from build123d import *

# Parameters (mm, degrees)
SKETCH1_W           = 55
SKETCH1_H           = 22
BOSS_EXTRUDE1_DEPTH = 18
CUT_EXTRUDE2_START  = -55
CUT_EXTRUDE2_DEPTH  = 55
SKETCH5_W           = 50
SKETCH5_H           = 17
CUT_EXTRUDE3_DEPTH  = 10
FILLET1_R           = 2.5
CUT_EXTRUDE4_DEPTH  = 3
SKETCH8_W           = 5.5
SKETCH8_H           = 1.5
CUT_EXTRUDE5_DEPTH  = 32


# Read off the part's stored shape, not the designer's step: Cut-Extrude2
with BuildPart() as part:
    # Sketch1 → Boss-Extrude1 (new body)
    with BuildSketch(Plane.XY):
        with Locations((-16.417297699, 9.516109874)):
            Rectangle(SKETCH1_W, SKETCH1_H)
    extrude(amount=BOSS_EXTRUDE1_DEPTH)

    # Cut-Extrude2 outline → Cut-Extrude2 (cut)
    with BuildSketch(Plane(origin=(11.082702301, 0, 0), x_dir=(0, 0, -1), z_dir=(1, 0, 0)).offset(CUT_EXTRUDE2_START)):
        with BuildLine():
            add(Edge.make_bspline(
                [(0, 1.8942341), (-9.999457611, 9.516109874), (0, 17.137985647)],
                knots=[0, 0, 0, 1, 1, 1], degree=2))
            Line((0, 1.8942341), (0, 17.137985647))
        make_face()
    extrude(amount=CUT_EXTRUDE2_DEPTH, mode=Mode.SUBTRACT)

    # Sketch5 → Cut-Extrude3 (cut)
    with BuildSketch(Plane(origin=(0, 0, 0), x_dir=(-1, 0, 0), z_dir=(0, 0, -1))):
        with Locations((16.417297699, 9.516109874)):
            Rectangle(SKETCH5_W, SKETCH5_H)
    extrude(amount=-CUT_EXTRUDE3_DEPTH, mode=Mode.SUBTRACT)

    # Fillet1
    fillet1_edges = [part.edges().sort_by_distance(p)[0] for p in [
        (11.082702301, 9.516109874, 18),
        (-16.417297699, 20.516109874, 18),
        (-43.917297699, 9.516109874, 18),
        (-16.417297699, -1.483890126, 18),
    ]]
    fillet(fillet1_edges, radius=FILLET1_R)

    # Sketch7 → Cut-Extrude4 (cut)
    with BuildSketch(Plane.XY.offset(18)):
        with BuildLine():
            Line((-39.308664902, 14.016109874), (-20.917297699, 14.016109874))
            Line((-20.917297699, 14.016109874), (-20.917297699, 18.016109874))
            ThreePointArc((-20.917297699, 18.016109874), (-16.417297699, 22.516109874), (-11.917297699, 18.016109874))
            Line((-11.917297699, 18.016109874), (-11.917297699, 14.016109874))
            Line((-11.917297699, 14.016109874), (6.474069505, 14.016109874))
            ThreePointArc((6.474069505, 14.016109874), (10.974069505, 9.516109874), (6.474069505, 5.016109874))
            Line((6.474069505, 5.016109874), (-11.917297699, 5.016109874))
            Line((-11.917297699, 5.016109874), (-11.917297699, 1.016109874))
            ThreePointArc((-11.917297699, 1.016109874), (-16.417297699, -3.483890126), (-20.917297699, 1.016109874))
            Line((-20.917297699, 1.016109874), (-20.917297699, 5.016109874))
            Line((-20.917297699, 5.016109874), (-39.308664902, 5.016109874))
            ThreePointArc((-39.308664902, 5.016109874), (-43.808664902, 9.516109874), (-39.308664902, 14.016109874))
        make_face()
    extrude(amount=-CUT_EXTRUDE4_DEPTH, mode=Mode.SUBTRACT)

    # Sketch8 → Cut-Extrude5 (cut)
    with BuildSketch(Plane(origin=(0, 20.516109874, 0), x_dir=(1, 0, 0), z_dir=(0, 1, 0))):
        with Locations((-37.042297699, -13.165280764)):
            Rectangle(SKETCH8_W, SKETCH8_H)
        with Locations((-7.250631032, -13.165280764)):
            Rectangle(SKETCH8_W, SKETCH8_H)
        with Locations((4.207702301, -13.165280764)):
            Rectangle(SKETCH8_W, SKETCH8_H)
        with Locations((-25.583964365, -13.165280764)):
            Rectangle(SKETCH8_W, SKETCH8_H)
    extrude(amount=-CUT_EXTRUDE5_DEPTH, mode=Mode.SUBTRACT)


solid = part.part
Could you check a few things on this model? Use its own coordinates, in mm. A direction names the side the tool comes from. Give positions to 0.01 mm unless a question says otherwise; leave off trailing zeros. Order: outer loops, then holes, each group sorted by start corner. A loop starts at its lowest first (then second) coordinate and runs counter-clockwise, first axis right, second up.
1. Thinking about a two-plate mould opening in X: for faces 5 (the flat face through (-20.917, 16, 17)), 6 (the cylindrical face through (-43.48, 7.23, 16.91)), 7 (the flat face through (11.083, 9, 9)), 8 (the cylindrical face through (-0.63, -0.73, 17.29)), which applies, +X half, -X half, draft (parallel to the pull), parting line (faces both ways), or undercut?
Answers below:
face 5: undercut
face 6: -X half
face 7: +X half
face 8: draft
2. I need wall thicknesses on L1, parallel to Z at x = -28, y = 6.5; L2, parallel to Y at x = 8, z = 4.75; L3, parallel to X at y = 9, z = 7. Which ranges of each line are inside material? Lowest first, please.
Answers below:
L1: z = 10 to 12.42, 13.92 to 15
L2: y = -1.48 to 1.02, 18.02 to 20.52
L3: x = -43.92 to -41.42, 8.58 to 11.08
3. Suppose I cut it at A-A (x = 2.5). Write out the boundary of the cut face in (y, z).
Answers below:
outline: (-1.48, 0) - (1.02, 0) - (1.02, 10) - (18.02, 10) - (18.02, 0) - (20.52, 0) - (20.52, 12.42) - (-1.48, 12.42) - close; (-1.48, 13.92) - (20.52, 13.92) - (20.52, 15.5) arc R2.5 ccw to (18.02, 18) - (14.02, 18) - (14.02, 15) - (5.02, 15) - (5.02, 18) - (1.02, 18) arc R2.5 ccw to (-1.48, 15.5) - close
4. Which directions (+Z, -Z, +X, -X, +Y, -Y) give clear straight access to the entire face, cutting with the end or side of a thin tool? Please do faces 1 (the flat face through (-37, 10, 12.415)), 2 (the flat face through (8.583, 9, 6)), 3 (the flat face through (-2, 16, 18)), 4 (the flat face through (-11.917, 3, 17)).
Answers below:
face 1: +Y, -Y
face 2: -Z
face 3: +Z, +X, -X, +Y, -Y
face 4: +Z
5. For pin 1 (3.5 mm diameter, centred on x = -1.5, z = 17, fed in from +Y); pin 2 (2.5 mm diameter, centred on y = 17, z = 17, fed in from +X); pin 3 (5 mm diameter, centred on x = -10.5, y = 8, fed in from -Z); pin 4 (1.6 mm diameter, centred on x = -26.5, y = 12, fed in from +Z), each with a flat end and sliding along its axis, tell me the tip position at first contact or that it passes through.
Answers below:
pin 1: stops at y = 20.52
pin 2: stops at x = 11.07
pin 3: stops at z = 10
pin 4: stops at z = 15
6. Suppose I cut it at B-B (z = 9.25). Write out the boundary of the cut face in (x, y), plus the area to 3 significant figures.
Answers below:
outline: (-43.92, -1.48) - (11.08, -1.48) - (11.08, 20.52) - (-43.92, 20.52) - close; hole (-41.42, 1.02) - (8.58, 1.02) - (8.58, 18.02) - (-41.42, 18.02) - close
area: 360 mm2
7. Suppose I cut it at D-D (y = 6.5). State how many separate pieces and enclosed holes the cut face has, plus the area to 3 significant figures.
Answers below:
separate pieces: 1
enclosed holes: 4
area: 276 mm2
8. Suppose I cut it at C-C (x = -18). Write out the boundary of the cut face in (y, z), plus the area to 3 significant figures.
Answers below:
outline: (-1.48, 0) - (1.02, 0) - (1.02, 10) - (18.02, 10) - (18.02, 0) - (20.52, 0) - (20.52, 15) - (-1.48, 15) - close
area: 160 mm2
